Source: CAD feature listing. Evaluate the final solid. Frame: model axes, mm. A direction names the side the tool comes from. Round coordinates to 2 decimals unless told otherwise and drop trailing zeros. Order: outer loops, then holes, each group sorted by start corner. A loop starts at its lowest first (then second) coordinate and runs counter-clockwise, first axis right, second up. Notation, with made-up numbers: (66, -7.75) -> (101, -7.75) arc R22 cw to (101, 12.25) -> close; hole circle Ø7 at (38, -9). An arc over 180 degrees is marked (long way). Answer as CSV lines item,"result".
from build123d import *

# Parameters (mm, degrees)
SKETCH1_W           = 6
SKETCH1_H           = 8
BOSS_EXTRUDE1_DEPTH = 15
CUT_EXTRUDE2_DEPTH  = 15
SKETCH3_W           = 1.55025835
SKETCH3_H           = 0.5
SKETCH3_W_2         = 0.44974165
SKETCH3_W_3         = 1
SKETCH3_W_4         = 0.511037603
SKETCH3_W_5         = 1.033479195
SKETCH3_W_6         = 0.476588297
SKETCH3_W_7         = 0.523411703
SKETCH3_W_8         = 0.489932508
CUT_EXTRUDE3_DEPTH  = 15


with BuildPart() as part:
    # Sketch1 → Boss-Extrude1 (new body)
    with BuildSketch(Plane(origin=(0, 0, 0), x_dir=(1, 0, 0), z_dir=(0, 1, 0))):
        with Locations((3, 4)):
            Rectangle(SKETCH1_W, SKETCH1_H)
    extrude(amount=BOSS_EXTRUDE1_DEPTH)

    # Sketch2 → Cut-Extrude2 (cut)
    with BuildSketch(Plane(origin=(0, 15, 0), x_dir=(1, 0, 0), z_dir=(0, 1, 0))):
        with BuildLine():
            Line((4, 0), (2, 0))
            Line((2, 0), (2, 1.894320503))
            ThreePointArc((2, 1.894320503), (3, 6.331069742), (4, 1.894320503))
            Line((4, 1.894320503), (4, 0))
        make_face()
    extrude(amount=-CUT_EXTRUDE2_DEPTH, mode=Mode.SUBTRACT)

    # Sketch3 → Cut-Extrude3 (cut)
    with BuildSketch(Plane(origin=(0, 15, 0), x_dir=(1, 0, 0), z_dir=(0, 1, 0))):
        with Locations((5.224870825, 7.25)):
            Rectangle(SKETCH3_W, SKETCH3_H)
        with Locations((4.224870825, 7.25)):
            Rectangle(SKETCH3_W_2, SKETCH3_H)
        with Locations((5.5, 6.25)):
            Rectangle(SKETCH3_W_3, SKETCH3_H)
        with Locations((5.744481199, 5.25)):
            Rectangle(SKETCH3_W_4, SKETCH3_H)
        with Locations((5.744481199, 4.25)):
            Rectangle(SKETCH3_W_4, SKETCH3_H)
        with Locations((5.744481199, 3.25)):
            Rectangle(SKETCH3_W_4, SKETCH3_H)
        with Locations((5.744481199, 2.25)):
            Rectangle(SKETCH3_W_4, SKETCH3_H)
        with Locations((5.5, 1.25)):
            Rectangle(SKETCH3_W_3, SKETCH3_H)
        with Locations((5.224870825, 0.517991792)):
            Rectangle(SKETCH3_W, SKETCH3_H)
        with Locations((0.993327895, 0.517991792)):
            Rectangle(SKETCH3_W_5, SKETCH3_H)
        with Locations((0.238294149, 0.517991792)):
            Rectangle(SKETCH3_W_6, SKETCH3_H)
        with Locations((0.238294149, 1.25)):
            Rectangle(SKETCH3_W_6, SKETCH3_H)
        with Locations((0.738294149, 1.25)):
            Rectangle(SKETCH3_W_7, SKETCH3_H)
        with Locations((0.238294149, 2.25)):
            Rectangle(SKETCH3_W_6, SKETCH3_H)
        with Locations((0.238294149, 3.25)):
            Rectangle(SKETCH3_W_6, SKETCH3_H)
        with Locations((0.238294149, 4.25)):
            Rectangle(SKETCH3_W_6, SKETCH3_H)
        with Locations((0.238294149, 5.25)):
            Rectangle(SKETCH3_W_6, SKETCH3_H)
        with Locations((0.238294149, 6.25)):
            Rectangle(SKETCH3_W_6, SKETCH3_H)
        with Locations((0.993327895, 7.25)):
            Rectangle(SKETCH3_W_5, SKETCH3_H)
        with Locations((0.238294149, 7.25)):
            Rectangle(SKETCH3_W_6, SKETCH3_H)
        with Locations((1.755033746, 7.25)):
            Rectangle(SKETCH3_W_8, SKETCH3_H)
        with Locations((0.738294149, 6.25)):
            Rectangle(SKETCH3_W_7, SKETCH3_H)
    extrude(amount=-CUT_EXTRUDE3_DEPTH, mode=Mode.SUBTRACT)


solid = part.part
1. Reachability of faces 1 (the cylindrical face through (2.91, 7.6, -6.33)), 2 (the flat face through (4, 8, -1)), 3 (the flat face through (5.5, 7.6, -1)), 4 (the flat face through (1, 8, -7)) from +Z, -Z, +X, -X, +Y, -Y: full face, straight path, thin tool, end or side. Return the list, or none.
Results below:
face 1,"+Y, -Y"
face 2,"+Z, +Y, -Y"
face 3,"+X, +Y, -Y"
face 4,"-X, +Y, -Y"
2. Section query A-A on z = -1.75. Return loops of the section in (x, y).
Results below:
outline,"(0, 0) -> (2, 0) -> (2, 15) -> (0, 15) -> close; (4, 0) -> (6, 0) -> (6, 15) -> (4, 15) -> close"
3. Mould query, pull axis Z, two halves, no side actions, for faces 5 (the flat face through (1, 7, 0)), 6 (the flat face through (5, 8, -0.768)), 7 (the flat face through (3, 0, -7)). Classes: released by +Z, released by -Z, zero draft, split by the parting line, or undercut.
Results below:
face 5,"released by +Z"
face 6,"undercut"
face 7,"zero draft"
4. Section query B-B on x = 3. Return loops of the section in (y, z), and give its area (3 significant figures).
Results below:
outline,"(0, -8) -> (15, -8) -> (15, -6.33) -> (0, -6.33) -> close"
area,"25.0 mm2"
5. Pin query (flat end, axial travel): pin 1 (3 mm diameter, centred on x = 4.5, z = -5, fed in from +Y). Return the tip coordinate at first contact, or that it passes through.
Results below:
pin 1,"y = 15"
6. Section query D-D on z = -3.25. Return loops of the section in (x, y).
Results below:
outline,"(0.48, 0) -> (0.79, 0) -> (0.79, 15) -> (0.48, 15) -> close; (5.21, 0) -> (5.49, 0) -> (5.49, 15) -> (5.21, 15) -> close"
7. Section query C-C on x = 5.75. Give the number of separate pieces and of enclosed holes in the cut face, and give its area (3 significant figures).
Results below:
separate pieces,"9"
enclosed holes,"0"
area,"60.0 mm2"
8. Line query: L1, parallel to X at y = 2.75, z = -0.5; L2, parallel to Z at x = 3, y = 4.75; L3, parallel to Z at x = 3.75, y = 11. Output: solid intervals per line, ascending. Write a range as [from, to].
Results below:
L1,"[1.51, 2], [4, 4.45]"
L2,"[-8, -6.33]"
L3,"[-8, -6.21]"
